```python
from build123d import *

# Parameters (mm, degrees)
SKETCH1_W           = 15
SKETCH1_H           = 11
BOSS_EXTRUDE1_DEPTH = 21.5
SKETCH2_W           = 10
SKETCH2_H           = 11
BOSS_EXTRUDE2_DEPTH = 9
SKETCH3_R           = 2
BOSS_EXTRUDE3_DEPTH = 0.7
SKETCH4_R           = 1.5
BOSS_EXTRUDE4_DEPTH = 10
CUT_EXTRUDE1_DEPTH  = 10
SKETCH6_R           = 0.7
SKETCH6_R_2         = 1
CUT_EXTRUDE2_DEPTH  = 3
SKETCH7_W           = 7.64
SKETCH7_H           = 11
BOSS_EXTRUDE5_DEPTH = 10.16
SKETCH8_W           = 5
SKETCH8_H           = 13.3399974
CUT_EXTRUDE3_DEPTH  = 11


with BuildPart() as part:
    # Sketch1 → Boss-Extrude1 (new body)
    with BuildSketch(Plane.XY):
        Rectangle(SKETCH1_W, SKETCH1_H)
    extrude(amount=BOSS_EXTRUDE1_DEPTH)

    # Sketch2 → Boss-Extrude2 (add)
    with BuildSketch(Plane.XY.offset(21.5)):
        with Locations((2.5, 0)):
            Rectangle(SKETCH2_W, SKETCH2_H)
    extrude(amount=BOSS_EXTRUDE2_DEPTH)

    # Sketch3 → Boss-Extrude3 (add)
    with BuildSketch(Plane.XY.offset(30.5)):
        with Locations((2.5, 0)):
            Circle(SKETCH3_R)
    extrude(amount=BOSS_EXTRUDE3_DEPTH)

    # Sketch4 → Boss-Extrude4 (add)
    with BuildSketch(Plane.XY.offset(31.2)):
        with Locations((2.5, 0)):
            Circle(SKETCH4_R)
    extrude(amount=BOSS_EXTRUDE4_DEPTH)

    # Sketch5 → Cut-Extrude1 (cut)
    with BuildSketch(Plane.XY.offset(41.2)):
        with BuildLine():
            Line((1.381966011, 1), (3.618033989, 1))
            ThreePointArc((3.618033989, 1), (2.5, 1.5), (1.381966011, 1))
        make_face()
    extrude(amount=-CUT_EXTRUDE1_DEPTH, mode=Mode.SUBTRACT)

    # Sketch6 → Cut-Extrude2 (cut)
    with BuildSketch(Plane.XY.offset(30.5)):
        with Locations((2.5, 4.5)):
            Circle(SKETCH6_R)
        with Locations((2.5, -4.5)):
            Circle(SKETCH6_R)
        with Locations((4.75, -3.75)):
            Circle(SKETCH6_R_2)
        with Locations((0.25, 3.75)):
            Circle(SKETCH6_R_2)
    extrude(amount=-CUT_EXTRUDE2_DEPTH, mode=Mode.SUBTRACT)

    # Sketch7 → Boss-Extrude5 (add)
    with BuildSketch(Plane.ZY.offset(7.5)):
        with Locations((3.82, 0)):
            Rectangle(SKETCH7_W, SKETCH7_H)
    extrude(amount=BOSS_EXTRUDE5_DEPTH)

    # Sketch8 → Cut-Extrude3 (cut)
    with BuildSketch(Plane.XZ.offset(5.5)):
        with Locations((-5, 14.8300013)):
            Rectangle(SKETCH8_W, SKETCH8_H)
    extrude(amount=-CUT_EXTRUDE3_DEPTH, mode=Mode.SUBTRACT)


solid = part.part
```
Here's how the part is built. I have some questions about the finished solid (model axes, mm). A direction names the side the tool comes from. Round coordinates to 2 decimals unless told otherwise and drop trailing zeros. Order: outer loops, then holes, each group sorted by start corner. A loop starts at its lowest first (then second) coordinate and runs counter-clockwise, first axis right, second up. Notation, with made-up numbers: (39.25, 20.25) -> (83.25, 20.25) arc R21 ccw to (83.25, 52.25) -> close; hole circle Ø5 at (5.5, -21). An arc over 180 degrees is marked (long way). Use a Markdown table: item, result. Add a question column.
(1) Suppose I cut it at D-D, the plane z = 22. Please give me the cut outline in (x, y).
(2) For pin 1 Ø5.5 at (y, z) = (2.5, 22.5) entering from -X; pin 2 Ø1.1 at (x, y) = (2.5, -4.5) entering from +Z; pin 3 Ø4 at (y, z) = (-2, 8.5) entering from -X; pin 4 Ø3 at (x, y) = (-14.5, -0.5) entering from +Z, each with a flat end and sliding along its axis, tell me the tip position at first contact or that it passes through.
(3) Suppose I cut it at B-B, the plane z = 28.5. Please give me the cut outline in (x, y).
(4) If we mould it in two halves opening along Y, with no side actions, what happens to faces 5 (the face through (0, 0, 30.5)), 6 (the face through (4.013, -3.074, 29.021)), 7 (the face through (0, 4, 27.5)), 8 (the face through (1, 5.5, 12))? For each: released by +Y, released by -Y, zero draft, split by the parting line, or undercut.
(5) I need wall thicknesses on line 1 along Y through (x, z) = (2.5, 29.65); line 2 along Y through (x, z) = (0.25, 28.25); line 3 along Y through (x, z) = (4.75, 29). Which ranges of each line are inside material? Lowest first, please.
(6) For faces 1 (the face through (7.5, 0, 15)), 2 (the face through (2, 1, 36)), 3 (the face through (-2.5, 0, 19)), 4 (the face through (2.823, -5.121, 29.021)), which set-ups out of +Z, -Z, +X, -X, +Y, -Y let a thin tool reach every point of the face, with its end or its side?
(7) Suppose I cut it at C-C, the plane x = -5.75. Please give me the cut outline in (y, z).
(8) Suppose I cut it at A-A, the plane y = 0. Please give me the cut outline in (x, z), and give its area (3 significant figures).
Verdict:
| question | item | result |
|---|---|---|
| 1 | outline | (-2.5, -5.5) -> (7.5, -5.5) -> (7.5, 5.5) -> (-2.5, 5.5) -> close |
| 2 | pin 1 | x = -2.5 |
| 2 | pin 2 | z = 27.5 |
| 2 | pin 3 | x = -17.66 |
| 2 | pin 4 | z = 7.64 |
| 3 | outline | (-2.5, -5.5) -> (7.5, -5.5) -> (7.5, 5.5) -> (-2.5, 5.5) -> close; hole circle Ø2 at (0.25, 3.75); hole circle Ø1.4 at (2.5, -4.5); hole circle Ø1.4 at (2.5, 4.5); hole circle Ø2 at (4.75, -3.75) |
| 4 | face 5 | zero draft |
| 4 | face 6 | undercut |
| 4 | face 7 | undercut |
| 4 | face 8 | released by +Y |
| 5 | line 1 | -5.5 to -5.2, -3.8 to 3.8, 5.2 to 5.5 |
| 5 | line 2 | -5.5 to 2.75, 4.75 to 5.5 |
| 5 | line 3 | -5.5 to -4.75, -2.75 to 5.5 |
| 6 | face 1 | +Z, -Z, +X, +Y, -Y |
| 6 | face 2 | +Z, +X, -X, +Y |
| 6 | face 3 | +Z, -X, +Y, -Y |
| 6 | face 4 | +Z |
| 7 | outline | (-5.5, 0) -> (5.5, 0) -> (5.5, 8.16) -> (-5.5, 8.16) -> close |
| 8 | outline | (-17.66, 0) -> (7.5, 0) -> (7.5, 30.5) -> (4.5, 30.5) -> (4.5, 31.2) -> (4, 31.2) -> (4, 41.2) -> (1, 41.2) -> (1, 31.2) -> (0.5, 31.2) -> (0.5, 30.5) -> (-2.5, 30.5) -> (-2.5, 8.16) -> (-7.5, 8.16) -> (-7.5, 7.64) -> (-17.66, 7.64) -> close |
| 8 | area | 456 mm2 |
